```python
from build123d import *

# Parameters (mm, degrees)
SKETCH1_R             = 7
BOSS_EXTRUDE1_DEPTH   = 38.63
SKETCH2_W             = 2.872896842
SKETCH2_H             = 13.203310437
BOSS_EXTRUDE2_DEPTH   = 3
SKETCH2_H_2           = 13.668710778
BOSS_EXTRUDE2_2_DEPTH = 3
SKETCH3_W             = 2.872896842
SKETCH3_H             = 13.668710778
SKETCH3_H_2           = 13.203310437
BOSS_EXTRUDE3_DEPTH   = 10


with BuildPart() as part:
    # Sketch1 → Boss-Extrude1 (new body)
    with BuildSketch(Plane.XY):
        Circle(SKETCH1_R)
    extrude(amount=BOSS_EXTRUDE1_DEPTH)



with BuildPart() as body_2:
    # Sketch2 → Boss-Extrude2 (new body)
    with BuildSketch(Plane(origin=(-4.013864175, -5.73488399, 0), x_dir=(-0.819269141, 0.573409168, 0), z_dir=(-0.573409168, -0.819269141, 0))):
        with Locations((0.171883624, -6.601655219)):
            Rectangle(SKETCH2_W, SKETCH2_H)
    extrude(amount=BOSS_EXTRUDE2_DEPTH)


with BuildPart() as body_3:
    # Sketch2 → Boss-Extrude2 2 (new body)
    with BuildSketch(Plane(origin=(-4.013864175, -5.73488399, 0), x_dir=(-0.819269141, 0.573409168, 0), z_dir=(-0.573409168, -0.819269141, 0))):
        with Locations((0.171883624, -31.795644611)):
            Rectangle(SKETCH2_W, SKETCH2_H_2)
    extrude(amount=BOSS_EXTRUDE2_2_DEPTH)


with BuildPart() as part_1:
    add(part.part)

    add(body_2.part)  # Boss-Extrude3 merges body 2

    add(body_3.part)  # Boss-Extrude3 merges body 3
    # Sketch3 → Boss-Extrude3 (add)
    with BuildSketch(Plane(origin=(-4.013864175, -5.73488399, 0), x_dir=(0.819269141, -0.573409168, 0), z_dir=(0.573409168, 0.819269141, 0))):
        with Locations((-0.171883624, -31.795644611)):
            Rectangle(SKETCH3_W, SKETCH3_H)
        with Locations((-0.171883624, -6.601655219)):
            Rectangle(SKETCH3_W, SKETCH3_H_2)
    extrude(amount=BOSS_EXTRUDE3_DEPTH)


solid = part_1.part
```
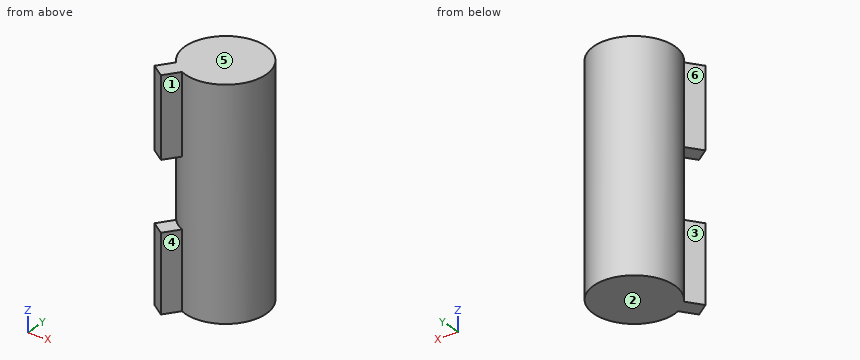
Check sheet for the modelled part. Datum: model origin and axes. Units: mm. Face numbers are marked on the shaded views. A direction names the side the tool comes from. Round coordinates to 2 decimals unless told otherwise and drop trailing zeros. Loops run counter-clockwise (first coordinate to the right, second up) from the corner with the lowest first, then second, coordinate; pieces in that order, holes last. Notation, with made-up numbers: (-12, 12) - (16, 12) arc R21 cw to (16, 26) - close; hole circle Ø4 at (84, 63.5). An arc over 180 degrees is marked (long way). Write item = value, one per line. Start each with the question number.
Q1. Thickness scan on L1, parallel to Y at x = 0, z = 2; L2, parallel to Y at x = -6, z = 26.5; L3, parallel to X at y = -0.75, z = 22.5. Record the ranges inside material, lowest first.
Q2. Section check B-B (x = -5.75). Record the boundary of the cut face in (y, z), plus the area to 3 significant figures.
Q3. Release check for a two-part mould opening along Y. For the marked faces 4, 5 and 6 record: pulls with the +Y half, pulls with the -Y half, needs draft (parallel to the pull), parting line crosses it, or undercut.
Q4. Section check A-A (y = -6). Record the boundary of the cut face in (x, z).
Q5. Section check C-C (x = 0). Record the boundary of the cut face in (y, z), plus the area to 3 significant figures.
Q6. Access from +Z, -Z, +X, -X, +Y, -Y to the whole of each face (thin tool, end or side, straight path). Record for the marked faces 1, 2 and 3.
Q7. Section check D-D (z = 23.5). Record the boundary of the cut face in (x, y), plus the area to 3 significant figures.
Q8. Depth check by flat-ended pin: P1, Ø5, axis at y = -2.5, z = 7, coming from the +X side; P2, Ø5, axis at x = 1.5, z = 28, coming from the -Y side; P3, Ø8, axis at x = 0, z = 34, coming from the -Y side; P4, Ø2, axis at x = 2.5, z = 8.5, coming from the +Y side. Enter the tip coordinate at first touch or a pass-through.
Derived:
q1.L1 = -7 to 7
q1.L2 = -8.01 to -5.77, -3.61 to 3.61
q1.L3 = -6.96 to 6.96
q2.outline = (-8.18, 0) - (-5.41, 0) - (-5.41, 13.2) - (-8.18, 13.2) - close; (-8.18, 24.96) - (-5.41, 24.96) - (-5.41, 38.63) - (-8.18, 38.63) - close; (-3.99, 0) - (3.99, 0) - (3.99, 38.63) - (-3.99, 38.63) - close
q2.area = 383 mm^2
q3.face_4 = pulls with the -Y half
q3.face_5 = needs draft
q3.face_6 = undercut
q4.outline = (-6.16, 0) - (3.61, 0) - (3.61, 38.63) - (-6.16, 38.63) - (-6.16, 24.96) - (-3.61, 24.96) - (-3.61, 13.2) - (-6.16, 13.2) - close
q5.outline = (-7, 0) - (7, 0) - (7, 38.63) - (-7, 38.63) - close
q5.area = 541 mm^2
q6.face_1 = +Z, -Z, -Y
q6.face_2 = -Z, +X, -X, +Y, -Y
q6.face_3 = +Z, -Z, -X
q7.outline = circle Ø14 at (0, 0)
q7.area = 154 mm^2
q8.P1 = 7
q8.P2 = -7
q8.P3 = -7.92
q8.P4 = 6.84
